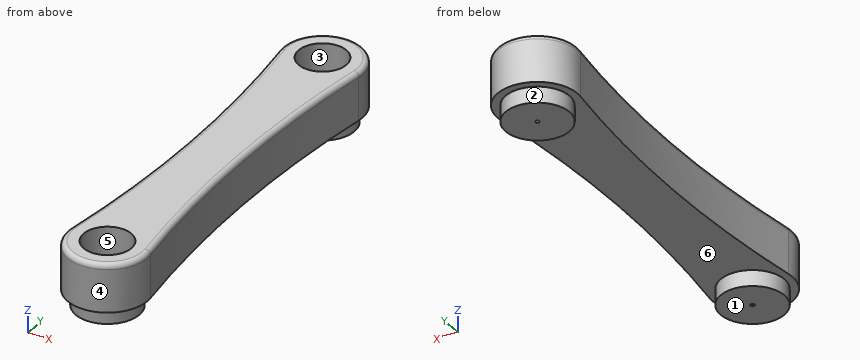
Autodesk Inventor part; units mm, degrees
ref_plane "YZ Plane" through (0, 0, 0) normal (1, 0, 0) x (0, 1, 0)
ref_plane "XZ Plane" through (0, 0, 0) normal (0, 1, 0) x (-1, 0, 0)
ref_plane "XY Plane" through (0, 0, 0) normal (0, 0, 1) x (1, 0, 0)
sketch "Sketch1" plane through (0, 0, 0) normal (0, 0, 1) x (1, 0, 0)
  circle A0 centre (0, 0) radius 50
  circle A1 centre (0, 450) radius 50
  arc A2 (49.4865, 442.8526) -> (49.4865, 7.1474) centre (1557.8354, 225) ccw
  arc A3 (-49.4865, 7.1474) -> (-49.4865, 442.8526) centre (-1557.8354, 225) ccw
  dimension "d0" = 100
  dimension "d1" = 450
  dimension "d2" = 1524
extrude "Extrusion1" add sketch "Sketch1" along normal blind 60
fillet "Fillet1" radius 6.35 4 edges at (-33.8354, 225, 60) (0, -50, 60) (33.8354, 225, 60) (0, 500, 60)
sketch "Sketch2" plane through (0, 0, 0) normal (0, 0, -1) x (-1, 0, 0)
  circle A0 centre (0, 450) radius 40
  circle A1 centre (0, 0) radius 40
  arc A2 (49.4865, 442.8526) -> (49.4865, 7.1474) centre (1557.8354, 225) ccw
  arc A3 (49.4865, 442.8526) -> (-49.4865, 442.8526) centre (0, 450) ccw
  arc A4 (-49.4865, 7.1474) -> (-49.4865, 442.8526) centre (-1557.8354, 225) ccw
  arc A5 (-49.4865, 7.1474) -> (49.4865, 7.1474) centre (0, 0) ccw
  dimension "d6" = 80
extrude "Extrusion2" add sketch "Sketch2" along normal blind 20 contours A0 | A1
sketch "Sketch3" plane through (0, 0, 60) normal (0, 0, 1) x (1, 0, 0)
  circle A0 centre (0, 0) radius 30
  arc A1 (-43.2017, 6.2397) -> (-43.2017, 443.7603) centre (-1557.8354, 225) ccw
  arc A2 (-43.2017, 6.2397) -> (43.2017, 6.2397) centre (0, 0) ccw
  arc A3 (43.2017, 443.7603) -> (43.2017, 6.2397) centre (1557.8354, 225) ccw
  arc A4 (43.2017, 443.7603) -> (-43.2017, 443.7603) centre (0, 450) ccw
  circle A5 centre (0, 450) radius 30
  dimension "d9" = 60
extrude "Extrusion3" cut sketch "Sketch3" against normal blind 70 contours A0 | A5
sketch "Sketch4" plane through (0, 450, -10) normal (0, 0, 1) x (1, 0, 0)
  circle A0 centre (0, 0) radius 30
  circle A1 centre (0, -450) radius 30
  circle A2 centre (0, 0) radius 2.5
  circle A3 centre (0, -450) radius 2.5
  dimension "d12" = 5
extrude "Extrusion4" cut sketch "Sketch4" against normal through all contours A2 | A3
properties part number "Robot_arm_1"
For this review, take the finished solid that the model builds, in its own axes (mm). Face numbers are marked on the shaded views. A direction names the side the tool comes from. Coordinates: 2 decimals unless noted, no trailing zeros. Loops run counter-clockwise (first coordinate to the right, second up) from the corner with the lowest first, then second, coordinate; pieces in that order, holes last.
1. For the marked faces 1, 2 and 3, list the 3-axis set-ups (+Z, -Z, +X, -X, +Y, -Y) from which the entire face can be reached by the end or side of a thin tool; tool diameter is ignored.
2. Add section A-A, the plane z = 44.5. Give the boundary of the cut face in (x, y).
3. Mouldability with a two-part tool opening along X and no side actions: class the marked faces 4, 5 and 6 as +X half, -X half, draft (parallel to the pull), parting line (faces both ways), or undercut.
4. For line 1 (Y direction, x = 0, z = 6); line 2 (Y direction, x = 0, z = -12); line 3 (Y direction, x = 1.5, z = -11), list the stretches that pass through material, from the lowest coordinate up.
5. Insertion check: P1, Ø1, axis at x = 13.5, y = 265.5, coming from the -Z side; P2, Ø18, axis at x = -10.5, y = -6, coming from the +Z side; P3, Ø4, axis at y = 425.5, z = 2, coming from the -X side. Each pin has a flat end and moves straight along its axis. Give the tip position at first contact, or say it passes through.
Result:
1. face 1: -Z, +X, -X, +Y, -Y
1. face 2: -Z
1. face 3: +Z
2. outline: (-49.49, 7.15) arc R50 ccw (long way) to (49.49, 7.15) arc R1524 cw to (49.49, 442.85) arc R50 ccw (long way) to (-49.49, 442.85) arc R1524 cw to start; hole circle Ø60 at (0, 0); hole circle Ø60 at (0, 450)
3. face 4: parting line
3. face 5: undercut
3. face 6: draft
4. line 1: y = -50 to -30, 30 to 420, 480 to 500
4. line 2: y = -40 to -2.5, 2.5 to 40, 410 to 447.5, 452.5 to 490
4. line 3: y = -39.97 to -2, 2 to 39.97, 410.03 to 448, 452 to 489.97
5. P1: stops at z = 0
5. P2: stops at z = -10
5. P3: stops at x = -47.35
